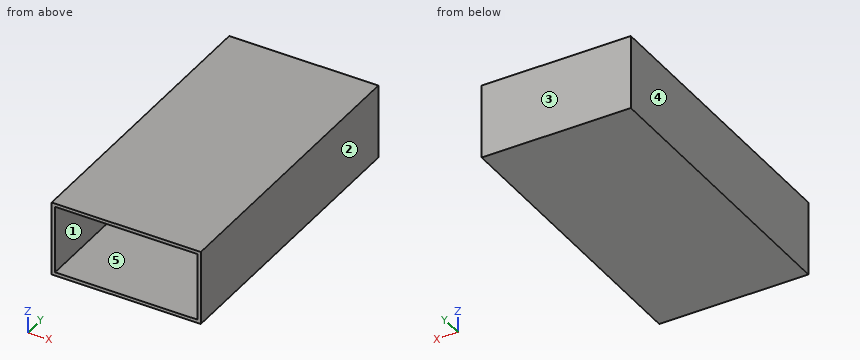
from build123d import *

# Parameters (mm, degrees)
F1_W     = 50.8
F1_H     = 25.4
F1_W_2   = 48.514
F1_H_2   = 23.114
F2_DEPTH = 101.6
F3_W     = 50.8
F3_H     = 25.4
F4_DEPTH = 22.86


with BuildPart() as f2:
    # F1 (on face) → F2 (new body)
    with BuildSketch(Plane.XZ):
        Rectangle(F1_W, F1_H)
        Rectangle(F1_W_2, F1_H_2, mode=Mode.SUBTRACT)
    extrude(amount=F2_DEPTH)

    # F3 (on Front) → F4 (join)
    with BuildSketch(Plane.XZ):
        Rectangle(F3_W, F3_H)
    extrude(amount=F4_DEPTH)


solid = f2.part
Read the model definition and answer for the solid it produces. Units are mm, in the model's axes. Face numbers are marked on the shaded views. A direction names the side the tool comes from. Round coordinates to 2 decimals unless told otherwise and drop trailing zeros. Order: outer loops, then holes, each group sorted by start corner. A loop starts at its lowest first (then second) coordinate and runs counter-clockwise, first axis right, second up. Notation, with made-up numbers: (50, 69.25) - (109, 69.25) arc R27 cw to (109, 85.25) - close; hole circle Ø10 at (29.5, 12.5). An arc over 180 degrees is marked (long way). Use one line per item in the form item = value. Start each with the question number.
(1) The part is cut by section A-A (x = 19). Give the vertices of the cut face in (y, z).
(2) A flat-ended cylindrical pin translates along its axis: pin 1 Ø8 at (x, z) = (17.5, 2) entering from -Y. Find the tip coordinate at first contact, or state that the pin passes through.
(3) Determine the mould class of the marked faces 3, 4 and 5 for opening direction X: +X half, -X half, draft (parallel to the pull), parting line (faces both ways), or undercut.
(4) The part is cut by section C-C (z = -1). Give the vertices of the cut face in (x, y).
(5) For the marked faces 1 and 2, determine the directions among +Z, -Z, +X, -X, +Y, -Y from which every point of the face is accessible in a straight line to the end or side of a thin tool.
(6) Find the intervals of material crossed by line 1 along X through (y, z) = (-71, 4); line 2 along Z through (x, y) = (4, -43.5); line 3 along Y through (x, z) = (-11.5, -6.5), in increasing order. Write a range as from..to.
(7) The part is cut by section B-B (y = -38). Give the vertices of the cut face in (x, z), then the cut area to 3 significant figures.
Checked values:
q1.outline = (-101.6, -12.7) - (0, -12.7) - (0, 12.7) - (-101.6, 12.7) - (-101.6, 11.56) - (-22.86, 11.56) - (-22.86, -11.56) - (-101.6, -11.56) - close
q2.pin_1 = -22.86
q3.face_3 = draft
q3.face_4 = -X half
q3.face_5 = undercut
q4.outline = (-25.4, -101.6) - (-24.26, -101.6) - (-24.26, -22.86) - (24.26, -22.86) - (24.26, -101.6) - (25.4, -101.6) - (25.4, 0) - (-25.4, 0) - close
q5.face_1 = -Y
q5.face_2 = +Z, -Z, +X, +Y, -Y
q6.line_1 = -25.4..-24.26, 24.26..25.4
q6.line_2 = -12.7..-11.56, 11.56..12.7
q6.line_3 = -22.86..0
q7.outline = (-25.4, -12.7) - (25.4, -12.7) - (25.4, 12.7) - (-25.4, 12.7) - close; hole (-24.26, -11.56) - (24.26, -11.56) - (24.26, 11.56) - (-24.26, 11.56) - close
q7.area = 169 mm^2
